Autodesk Inventor part; units mm, degrees
ref_plane "YZ Plane" through (0, 0, 0) normal (1, 0, 0) x (0, 1, 0)
ref_plane "XZ Plane" through (0, 0, 0) normal (0, 1, 0) x (-1, 0, 0)
ref_plane "XY Plane" through (0, 0, 0) normal (0, 0, 1) x (1, 0, 0)
sketch "Sketch1" plane through (0, 0, 0) normal (0, 0, 1) x (1, 0, 0)
  line L0 (-65, -219.5) -> (65, -219.5)
  line L1 (65, -219.5) -> (65, 219.5)
  line L2 (65, 219.5) -> (-65, 219.5)
  line L3 (-65, 219.5) -> (-65, -219.5)
  line L4 (-65, -219.5) -> (65, 219.5) construction
  line L5 (65, -219.5) -> (-65, 219.5) construction
  line L6 (58.93, -50) -> (62, -50)
  line L7 (62, -50) -> (62, 50)
  line L8 (62, 50) -> (58.93, 50)
  line L9 (58.93, 50) -> (58.93, -50)
  line L10 (58.93, -50) -> (62, 50) construction
  line L11 (62, -50) -> (58.93, 50) construction
  line L12 (0, 219.5) -> (0, -219.5)
  line L13 (-58.93, -50) -> (-62, -50)
  line L14 (-62, -50) -> (-62, 50)
  line L15 (-62, 50) -> (-58.93, 50)
  line L16 (-58.93, 50) -> (-58.93, -50)
  line L17 (-58.93, -50) -> (-62, 50) construction
  line L18 (-62, -50) -> (-58.93, 50) construction
  point P0 (0, 0)
  point P1 (60.465, 0)
  point P2 (62, 0)
  point P3 (-60.465, 0)
  point P4 (-62, 0)
  point P5 (0, 0)
  dimension "d0" = 130
  dimension "d1" = 439
  dimension "d2" = 3.07
  dimension "d3" = 100
  dimension "d4" = 3
extrude "Extrusion1" add sketch "Sketch1" along normal mid plane 5
sketch "Sketch2" plane through (0, 0, 2.5) normal (0, 0, 1) x (1, 0, 0)
  line L0 (-25, 219.5) -> (25, 219.5)
  line L1 (25, 219.5) -> (25, 224.5)
  line L2 (25, 224.5) -> (-25, 224.5)
  line L3 (-25, 224.5) -> (-25, 219.5)
  line L4 (-58.93, -50) -> (-58.93, 50)
  line L5 (-58.93, 0) -> (58.93, 0)
  line L6 (58.93, -50) -> (58.93, 50)
  line L7 (-25, -219.5) -> (25, -219.5)
  line L8 (25, -219.5) -> (25, -224.5)
  line L9 (25, -224.5) -> (-25, -224.5)
  line L10 (-25, -224.5) -> (-25, -219.5)
  point P0 (0, 0)
  point P1 (-65, 219.5)
  point P2 (0, 224.5)
  point P3 (0, -224.5)
  dimension "d7" = 50
  dimension "d8" = 5
extrude "Extrusion2" add sketch "Sketch2" against normal blind 5
Source: CAD feature listing. Evaluate the final solid. Frame: model axes, mm. Round coordinates to 2 decimals unless told otherwise and drop trailing zeros. Loops run counter-clockwise (first coordinate to the right, second up) from the corner with the lowest first, then second, coordinate; pieces in that order, holes last.
Q1. Section B-B, the plane z = 1.05. Return loops of the section in (x, y), plus the area to 3 significant figures.
Q2. First-contact query: P1, Ø0.9, axis at x = -60, z = -1, coming from the +Y side; P2, Ø2.5, axis at y = -223, z = 0.5, coming from the -X side; P3, Ø2.5, axis at y = 221.5, z = 0, coming from the +X side. Flat tips, straight axial feed; report the tip coordinate or a pass-through.
Q3. Ray query, line 1 (X direction, y = -47.5, z = 0.75); line 2 (Y direction, x = 37, z = 0.8). Return the intervals inside material, ascending.
Q4. Section C-C, the plane x = -54.5. Return loops of the section in (y, z).
Q5. Section A-A, the plane y = -34. Return loops of the section in (x, z), plus the area to 3 significant figures.
Solutions:
1. outline: (-65, -219.5) - (-25, -219.5) - (-25, -224.5) - (25, -224.5) - (25, -219.5) - (65, -219.5) - (65, 219.5) - (25, 219.5) - (25, 224.5) - (-25, 224.5) - (-25, 219.5) - (-65, 219.5) - close; hole (-62, -50) - (-58.93, -50) - (-58.93, 50) - (-62, 50) - close; hole (58.93, -50) - (62, -50) - (62, 50) - (58.93, 50) - close
1. area: 57,000 mm2
2. P1: stops at y = 219.5
2. P2: stops at x = -25
2. P3: stops at x = 25
3. line 1: x = -65 to -62, -58.93 to 58.93, 62 to 65
3. line 2: y = -219.5 to 219.5
4. outline: (-219.5, -2.5) - (219.5, -2.5) - (219.5, 2.5) - (-219.5, 2.5) - close
5. outline: (-65, -2.5) - (-62, -2.5) - (-62, 2.5) - (-65, 2.5) - close; (-58.93, -2.5) - (58.93, -2.5) - (58.93, 2.5) - (-58.93, 2.5) - close; (62, -2.5) - (65, -2.5) - (65, 2.5) - (62, 2.5) - close
5. area: 619 mm2
